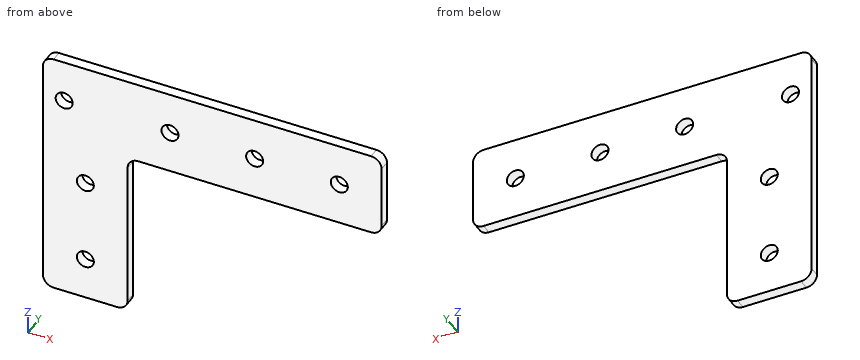
```python
from build123d import *

# Parameters (mm, degrees)
BOSS_EXTRUDE1_DEPTH    = 3.175
F_10_CLEARANCE_HOLE1_D = 5.1054
F_10_CLEARANCE_HOLE4_D = 5.1054
CUT_EXTRUDE1_DEPTH     = 128.039681301
FILLET1_R              = 3.175


with BuildPart() as part:
    # Sketch1 → Boss-Extrude1 (new body)
    with BuildSketch(Plane(origin=(0, 0, 0), x_dir=(1, 0, 0), z_dir=(0, 1, 0))):
        Polygon((0, 0), (0, 76.2), (25.4, 76.2), (101.6, 25.4), (101.6, 0), align=None)
    extrude(amount=BOSS_EXTRUDE1_DEPTH)

    # #10 Clearance Hole1 (through all)
    with Locations(Plane(origin=(0, 3.175, 0), x_dir=(1, 0, 0), z_dir=(0, 1, 0))):
        with Locations((88.9, 12.7), (12.7, 63.5), (12.7, 38.1), (38.1, 12.7), (63.5, 12.7)):
            Hole(F_10_CLEARANCE_HOLE1_D / 2)

    # #10 Clearance Hole4 (through all)
    with Locations(Plane(origin=(0, 3.175, 0), x_dir=(1, 0, 0), z_dir=(0, 1, 0))):
        with Locations((6.35, 12.7)):
            Hole(F_10_CLEARANCE_HOLE4_D / 2)

    # Sketch6 → Cut-Extrude1 (cut, through all)
    with BuildSketch(Plane(origin=(0, 3.175, 0), x_dir=(1, 0, 0), z_dir=(0, 1, 0))):
        Polygon((25.4, 76.2), (25.4, 25.4), (101.6, 25.4), align=None)
    extrude(amount=-CUT_EXTRUDE1_DEPTH, mode=Mode.SUBTRACT)

    # Fillet1
    fillet1_edges = [part.edges().sort_by_distance(p)[0] for p in [
        (25.4, 1.5875, -25.4),
        (0, 1.5875, 0),
        (0, 1.5875, -76.2),
        (25.4, 1.5875, -76.2),
        (101.6, 1.5875, -25.4),
        (101.6, 1.5875, 0),
    ]]
    fillet(fillet1_edges, radius=FILLET1_R)


solid = part.part
```
Geometry: final body of the model. Coordinates: model frame, mm. Round coordinates to 2 decimals unless told otherwise and drop trailing zeros. Loops run counter-clockwise (first coordinate to the right, second up) from the corner with the lowest first, then second, coordinate; pieces in that order, holes last. Notation, with made-up numbers: (4.5, 42) -> (11.5, 42) arc R23 ccw to (11.5, 72) -> close; hole circle Ø4 at (89.5, 35). An arc over 180 degrees is marked (long way). Use one line per item in the form item = value.
Item 1: Contact query for flat-ended pins moving along their axis: pin 1 Ø1.5 at (x, y) = (88, 2) entering from -Z; pin 2 Ø1.6 at (y, z) = (1, -40) entering from +X. Output: stop coordinate, or through.
Evaluation:
pin_1 = -25.4
pin_2 = 25.4
Item 2: Cut plane B-B on y = 1.6. Output: boundary loops of the cut face in (x, z) (3 decimals).
Evaluation:
outline = (0, -73.025) arc R3.175 ccw to (3.175, -76.2) -> (22.225, -76.2) arc R3.175 ccw to (25.4, -73.025) -> (25.4, -28.575) arc R3.175 cw to (28.575, -25.4) -> (98.425, -25.4) arc R3.175 ccw to (101.6, -22.225) -> (101.6, -3.175) arc R3.175 ccw to (98.425, 0) -> (3.175, 0) arc R3.175 ccw to (0, -3.175) -> close; hole circle Ø5.105 at (6.35, -12.7); hole circle Ø5.105 at (12.7, -63.5); hole circle Ø5.105 at (12.7, -38.1); hole circle Ø5.105 at (38.1, -12.7); hole circle Ø5.105 at (63.5, -12.7); hole circle Ø5.105 at (88.9, -12.7)
Item 3: Cut plane C-C on z = -63.5. Output: boundary loops of the cut face in (x, y) (3 decimals).
Evaluation:
outline = (0, 0) -> (10.147, 0) -> (10.147, 3.175) -> (0, 3.175) -> close; (15.253, 0) -> (25.4, 0) -> (25.4, 3.175) -> (15.253, 3.175) -> close
Item 4: Cut plane D-D on x = 38.1. Output: boundary loops of the cut face in (y, z) (3 decimals), then the cut area to 3 significant figures.
Evaluation:
outline = (0, -25.4) -> (3.175, -25.4) -> (3.175, -15.253) -> (0, -15.253) -> close; (0, -10.147) -> (3.175, -10.147) -> (3.175, 0) -> (0, 0) -> close
area = 64.4 mm2
Item 5: Material intervals for probe 1 along X at (y, z) = (1.8, -12.7); probe 2 along Z at (x, y) = (12.7, 1.55); probe 3 along Z at (x, y) = (88.9, 2.25), sorted ascending.
Evaluation:
probe_1 = 0 to 3.8, 8.9 to 35.55, 40.65 to 60.95, 66.05 to 86.35, 91.45 to 101.6
probe_2 = -76.2 to -66.05, -60.95 to -40.65, -35.55 to 0
probe_3 = -25.4 to -15.25, -10.15 to 0
Item 6: Cut plane A-A on x = 12.7. Output: boundary loops of the cut face in (y, z) (3 decimals).
Evaluation:
outline = (0, -76.2) -> (3.175, -76.2) -> (3.175, -66.053) -> (0, -66.053) -> close; (0, -60.947) -> (3.175, -60.947) -> (3.175, -40.653) -> (0, -40.653) -> close; (0, -35.547) -> (3.175, -35.547) -> (3.175, 0) -> (0, 0) -> close
